Source: CAD feature listing. Evaluate the final solid. Frame: model axes, mm. Face numbers are marked on the shaded views. Give positions to 0.01 mm unless a question says otherwise; leave off trailing zeros. Order: outer loops, then holes, each group sorted by start corner. A loop starts at its lowest first (then second) coordinate and runs counter-clockwise, first axis right, second up. Notation, with made-up numbers: M 36,32.25 L 80,32.25 A27 cw 80,49.25 Z; hole C 86.25,66 d10. An arc over 180 degrees is marked long. Answer in a Markdown table with one row per item. Add a question column.
(1) Material intervals for line 1 along X through (y, z) = (10.25, -5); line 2 along Y through (x, z) = (-7.5, 4); line 3 along Z through (x, y) = (-12, 5.25), sorted ascending.
(2) Section query C-C, the plane x = -8.75. Return loops of the section in (y, z), plus the area to 3 significant figures.
(3) Pin query (flat end, axial travel): P1, Ø2, axis at y = 11, z = -3.5, coming from the +X side; P2, Ø6, axis at x = -15.5, z = 1, coming from the +Y side; P3, Ø1, axis at x = -8.5, y = 0.5, coming from the +Z side. Return the tip coordinate at first contact, or that it passes through.
(4) Section query A-A, the plane z = -3. Return loops of the section in (x, y).
(5) Section query D-D, the plane z = 25.5. Return loops of the section in (x, y), plus the area to 3 significant figures.
(6) Section query B-B, the plane y = 11. Return loops of the section in (x, z), plus the area to 3 significant figures.
(7) Mould query, pull axis X, two halves, no side actions, for the marked faces 1 and 2. Classes: pulls with the +X half, pulls with the -X half, needs draft (parallel to the pull), parting line crosses it, or undercut.
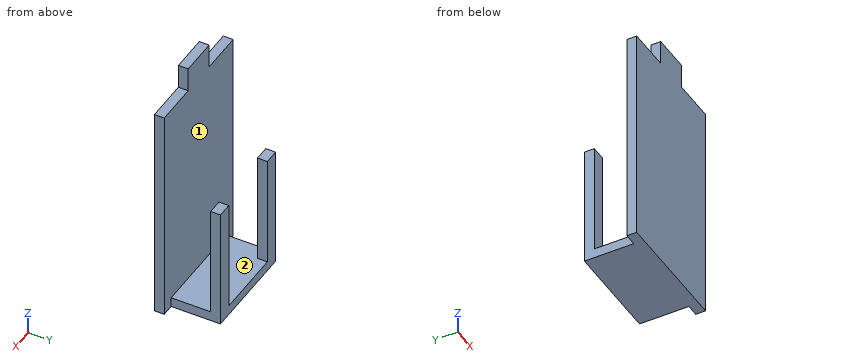
from build123d import *

# Parameters (mm, degrees)
SKETCH_1_W          = 25
SKETCH_1_H          = 50
EXTRUDE_1_DEPTH     = 2
SKETCH_3_W          = 20
SKETCH_3_H          = 2
EXTRUDE_2_DEPTH     = 10
SKETCH_4_W          = 20
SKETCH_4_H          = 2
EXTRUDE_3_DEPTH     = 23
SKETCH_5_W          = 14
SKETCH_5_H          = 23
CUT_EXTRUDE_1_DEPTH = 3
SKETCH_6_W          = 8.7
SKETCH_6_H          = 2
CUT_EXTRUDE_2_DEPTH = 5


with BuildPart() as part:
    # 草图1 → 凸台-拉伸1 (new body)
    with BuildSketch(Plane(origin=(0, 0, 0), x_dir=(1, 0, 0), z_dir=(0, 1, 0))):
        with Locations((-15.126272577, -4.709205827)):
            Rectangle(SKETCH_1_W, SKETCH_1_H)
    extrude(amount=EXTRUDE_1_DEPTH)

    # 草图3 → 凸台-拉伸2 (add)
    with BuildSketch(Plane(origin=(0, 2, 0), x_dir=(1, 0, 0), z_dir=(0, 1, 0))):
        with Locations((-15.126272577, 19.290794173)):
            Rectangle(SKETCH_3_W, SKETCH_3_H)
    extrude(amount=EXTRUDE_2_DEPTH)

    # 草图4 → 凸台-拉伸3 (add)
    with BuildSketch(Plane.XY.offset(-18.290794173)):
        with Locations((-15.126272577, 11)):
            Rectangle(SKETCH_4_W, SKETCH_4_H)
    extrude(amount=EXTRUDE_3_DEPTH)

    # 草图5 → 切除-拉伸1 (cut)
    with BuildSketch(Plane(origin=(0, 12, 0), x_dir=(1, 0, 0), z_dir=(0, 1, 0))):
        with Locations((-15.126272577, 6.790794173)):
            Rectangle(SKETCH_5_W, SKETCH_5_H)
    extrude(amount=-CUT_EXTRUDE_1_DEPTH, mode=Mode.SUBTRACT)

    # 草图6 → 切除-拉伸2 (cut)
    with BuildSketch(Plane.XY.offset(29.709205827)):
        with Locations((-6.976272577, 1)):
            Rectangle(SKETCH_6_W, SKETCH_6_H)
        with Locations((-23.276272577, 1)):
            Rectangle(SKETCH_6_W, SKETCH_6_H)
    extrude(amount=-CUT_EXTRUDE_2_DEPTH, mode=Mode.SUBTRACT)


solid = part.part
Values follow:
| question | item | result |
|---|---|---|
| 1 | line 1 | x = -25.13 to -22.13, -8.13 to -5.13 |
| 1 | line 2 | y = 0 to 2, 10 to 12 |
| 1 | line 3 | z = -20.29 to -18.29 |
| 2 | outline | M 0,-20.29 L 12,-20.29 L 12,-18.29 L 2,-18.29 L 2,24.71 L 0,24.71 Z |
| 2 | area | 110 mm² |
| 3 | P1 | stops at x = -5.13 |
| 3 | P2 | stops at y = 2 |
| 3 | P3 | stops at z = 24.71 |
| 4 | outline | M -27.63,0 L -2.63,0 L -2.63,2 L -27.63,2 Z; M -25.13,10 L -22.13,10 L -22.13,12 L -25.13,12 Z; M -8.13,10 L -5.13,10 L -5.13,12 L -8.13,12 Z |
| 5 | outline | M -18.93,0 L -11.33,0 L -11.33,2 L -18.93,2 Z |
| 5 | area | 15.2 mm² |
| 6 | outline | M -25.13,-20.29 L -5.13,-20.29 L -5.13,4.71 L -8.13,4.71 L -8.13,-18.29 L -22.13,-18.29 L -22.13,4.71 L -25.13,4.71 Z |
| 6 | area | 178 mm² |
| 7 | face 1 | needs draft |
| 7 | face 2 | undercut |
